Geometry: final body of the model. Coordinates: model frame, mm. Coordinates: 2 decimals unless noted, no trailing zeros. Order: outer loops, then holes, each group sorted by start corner. A loop starts at its lowest first (then second) coordinate and runs counter-clockwise, first axis right, second up. Notation, with made-up numbers: (25.5, 25) -> (75.5, 25) arc R22 ccw to (75.5, 32) -> close; hole circle Ø8 at (83, -32.75). An arc over 180 degrees is marked (long way). Answer in a Markdown table with one row per item. Add a question column.
1) Section query B-B on y = 63. Return the cut outline in (x, z).
2) Contact query for flat-ended pins moving along their axis: P1, Ø1.5, axis at y = 57.5, z = 2.5, coming from the +X side; P2, Ø3, axis at x = -2.48, y = 0, coming from the -Z side. Output: stop coordinate, or through.
3) Section query D-D on x = -31. Return the cut outline in (y, z), then the cut area to 3 significant figures.
4) Section query C-C on y = 0. Return the cut outline in (x, z).
5) Pull-direction query (Y, two-part tool) for faces 1 (the face through (-20.957, 0.481, 1.479)), 2 (the face through (-0.913, -0.651, 1.479)), 3 (the face through (-19.757, 33.27, 1.479)), 4 (the face through (-13, -4, 1)); classes: +Y half, -Y half, draft (parallel to the pull), parting line (faces both ways), or undercut.
6) Ray query, line 1 (Y direction, x = -23, z = 0.55); line 2 (X direction, y = 52.5, z = 2.2); line 3 (X direction, y = 20.5, z = 0.55). Return the intervals inside material, ascending. Write a range as from..to.
7) Section query A-A on z = 0.5. Return the cut outline in (x, y), then the cut area to 3 significant figures.
```python
from build123d import *

# Parameters (mm, degrees)
SKETCH_1_R      = 1.6
SKETCH_1_R_2    = 1.7
SKETCH_1_R_3    = 4
EXTRUDE_1_DEPTH = 3


with BuildPart() as part:
    # 草图1 → 凸台-拉伸1 (new body)
    # profile 1 of 3: a face of its own
    with BuildSketch(Plane.XY):
        with BuildLine():
            Line((-2.4830952, 4), (-22.4830952, 4))
            ThreePointArc((-22.4830952, 4), (-25.741324807, 2.320331836), (-26.263182143, -1.308030085))
            ThreePointArc((-26.263182143, -1.308030085), (-24.803427036, -3.258229607), (-22.4830952, -4))
            Line((-22.4830952, -4), (-2.4830952, -4))
            ThreePointArc((-2.4830952, -4), (1.041523919, -1.891311732), (0.849981545, 2.211469967))
            ThreePointArc((0.849981545, 2.211469967), (-0.591783468, 3.524619119), (-2.4830952, 4))
        make_face()
        with Locations((-22.4830952, 0)):
            Circle(SKETCH_1_R, mode=Mode.SUBTRACT)
        with Locations((-2.4830952, 0)):
            Circle(SKETCH_1_R_2, mode=Mode.SUBTRACT)
    # profile 2 of 3: a face of its own
    with BuildSketch(Plane.XY):
        with BuildLine():
            ThreePointArc((-26.263182143, -1.308030085), (-25.741324807, 2.320331836), (-22.4830952, 4))
            Line((-22.4830952, 4), (-2.4830952, 4))
            ThreePointArc((-2.4830952, 4), (-0.591783468, 3.524619119), (0.849981545, 2.211469967))
            Line((0.849981545, 2.211469967), (-40.950018455, 65.211469967))
            ThreePointArc((-40.950018455, 65.211469967), (-40.453453769, 64.154922729), (-40.2830952, 63))
            ThreePointArc((-40.2830952, 63), (-43.619901326, 59.055361374), (-48.063182143, 61.691969915))
            Line((-48.063182143, 61.691969915), (-26.263182143, -1.308030085))
        make_face()
    # profile 3 of 3: a face of its own
    with BuildSketch(Plane.XY):
        with Locations((-44.2830952, 63)):
            Circle(SKETCH_1_R_3)
        with Locations((-44.2830952, 63)):
            Circle(SKETCH_1_R_2, mode=Mode.SUBTRACT)
    extrude(amount=EXTRUDE_1_DEPTH)


solid = part.part
```
Result:
| question | item | result |
|---|---|---|
| 1 | outline | (-48.28, 0) -> (-45.98, 0) -> (-45.98, 3) -> (-48.28, 3) -> close; (-42.58, 0) -> (-39.48, 0) -> (-39.48, 3) -> (-42.58, 3) -> close |
| 2 | P1 | x = -35.34 |
| 2 | P2 | through |
| 3 | outline | (12.38, 0) -> (50.22, 0) -> (50.22, 3) -> (12.38, 3) -> close |
| 3 | area | 114 mm2 |
| 4 | outline | (-26.72, 0) -> (-24.08, 0) -> (-24.08, 3) -> (-26.72, 3) -> close; (-20.88, 0) -> (-4.18, 0) -> (-4.18, 3) -> (-20.88, 3) -> close; (-0.78, 0) -> (1.52, 0) -> (1.52, 3) -> (-0.78, 3) -> close |
| 5 | face 1 | undercut |
| 5 | face 2 | undercut |
| 5 | face 3 | +Y half |
| 5 | face 4 | -Y half |
| 6 | line 1 | -3.97..-1.51, 1.51..38.16 |
| 6 | line 2 | -44.88..-32.52 |
| 6 | line 3 | -33.81..-11.28 |
| 7 | outline | (-48.06, 61.69) -> (-26.26, -1.31) arc R4 ccw to (-22.48, -4) -> (-2.48, -4) arc R4 ccw to (0.85, 2.21) -> (-40.95, 65.21) arc R4 ccw to start; hole circle Ø3.4 at (-44.28, 63); hole circle Ø3.2 at (-22.48, 0); hole circle Ø3.4 at (-2.48, 0) |
| 7 | area | 1,300 mm2 |
